Part model, mm, in its own coordinate system. A direction names the side the tool comes from. Give positions to 0.01 mm unless a question says otherwise; leave off trailing zeros. Order: outer loops, then holes, each group sorted by start corner. A loop starts at its lowest first (then second) coordinate and runs counter-clockwise, first axis right, second up. Notation, with made-up numbers: (9.25, -29) - (27.25, -29) arc R23 ccw to (27.25, -3) - close; hole circle Ø4 at (86, 65.25). An arc over 180 degrees is marked (long way). One line per item, written item: value.
```python
from build123d import *

# Parameters (mm, degrees)
SKETCH1_W           = 914.4
SKETCH1_H           = 203.2
BOSS_EXTRUDE1_DEPTH = 12.7
SKETCH2_W           = 914.4
SKETCH2_H           = 152.4
BOSS_EXTRUDE2_DEPTH = 12.7
SKETCH3_W           = 31.75
SKETCH3_H           = 419.1
BOSS_EXTRUDE3_DEPTH = 31.75
BOSS_EXTRUDE4_START = -914.4
SKETCH3_2_W         = 31.75
SKETCH3_2_H         = 419.1
BOSS_EXTRUDE4_DEPTH = 31.75


with BuildPart() as part:
    # Sketch1 → Boss-Extrude1 (new body)
    with BuildSketch(Plane(origin=(0, 0, 0), x_dir=(1, 0, 0), z_dir=(0, 1, 0))):
        with Locations((457.2, 101.6)):
            Rectangle(SKETCH1_W, SKETCH1_H)
    extrude(amount=BOSS_EXTRUDE1_DEPTH)



with BuildPart() as body_2:
    # Sketch2 → Boss-Extrude2 (new body)
    with BuildSketch(Plane(origin=(0, 215.9, 0), x_dir=(1, 0, 0), z_dir=(0, 1, 0))):
        with Locations((457.2, 127)):
            Rectangle(SKETCH2_W, SKETCH2_H)
    extrude(amount=BOSS_EXTRUDE2_DEPTH)


with BuildPart() as part_1:
    add(part.part)

    add(body_2.part)  # Boss-Extrude3 merges body 2
    # Sketch3 → Boss-Extrude3 (add)
    with BuildSketch(Plane(origin=(914.4, 0, 0), x_dir=(0, 0, -1), z_dir=(1, 0, 0))):
        with Locations((187.325, 19.05)):
            Rectangle(SKETCH3_W, SKETCH3_H)
        Polygon((0, 12.7), (0, -190.5), (31.75, -190.5), (31.75, 12.7), (82.55, 228.6), (50.8, 228.6), align=None)
    extrude(amount=-BOSS_EXTRUDE3_DEPTH)

    # Sketch3<2> → Boss-Extrude4 (add)
    with BuildSketch(Plane(origin=(914.4, 0, 0), x_dir=(0, 0, -1), z_dir=(1, 0, 0)).offset(BOSS_EXTRUDE4_START)):
        with Locations((187.325, 19.05)):
            Rectangle(SKETCH3_2_W, SKETCH3_2_H)
        Polygon((0, 12.7), (0, -190.5), (31.75, -190.5), (31.75, 12.7), (82.55, 228.6), (50.8, 228.6), align=None)
    extrude(amount=BOSS_EXTRUDE4_DEPTH)


solid = part_1.part
```
1) Cut at C-C, the plane z = -16. Give the cut face in (x, y), then the cut area to 3 significant figures.
Outcome:
outline: (0, -190.5) - (31.75, -190.5) - (31.75, 0) - (882.65, 0) - (882.65, -190.5) - (914.4, -190.5) - (914.4, 80.7) - (882.65, 80.7) - (882.65, 12.7) - (31.75, 12.7) - (31.75, 80.7) - (0, 80.7) - close
area: 28,000 mm^2
2) Cut at B-B, the plane z = -105.5. Give the cut face in (x, y).
Outcome:
outline: (0, 0) - (914.4, 0) - (914.4, 12.7) - (0, 12.7) - close; (0, 215.9) - (914.4, 215.9) - (914.4, 228.6) - (0, 228.6) - close
3) Cut at A-A, the plane x = 205. Give the cut face in (y, z).
Outcome:
outline: (0, -203.2) - (12.7, -203.2) - (12.7, 0) - (0, 0) - close; (215.9, -203.2) - (228.6, -203.2) - (228.6, -50.8) - (215.9, -50.8) - close
4) Pin check, flat tips, straight feed: pin 1 (12 mm diameter, centred on x = 379, z = -34, fed in from +Y); pin 2 (4 mm diameter, centred on x = 225, z = -164.5, fed in from -Y); pin 3 (6 mm diameter, centred on y = -43, z = -165.5, fed in from -X). Stop position of each tip, or through.
Outcome:
pin 1: stops at y = 12.7
pin 2: stops at y = 0
pin 3: passes through
5) Drill centre lines: line 1 along X through (y, z) = (-52.5, -189.5); line 2 along Y through (x, z) = (567.5, -152.5); line 3 along Y through (x, z) = (779, -21). Where is each one in solid material? Low to high. Write a range as from..to.
Outcome:
line 1: x = 0..31.75, 882.65..914.4
line 2: y = 0..12.7, 215.9..228.6
line 3: y = 0..12.7
6) Cut at D-D, the plane y = 154. Give the cut face in (x, z), then the cut area to 3 significant figures.
Outcome:
outline: (0, -203.2) - (31.75, -203.2) - (31.75, -171.45) - (0, -171.45) - close; (0, -65) - (31.75, -65) - (31.75, -33.25) - (0, -33.25) - close; (882.65, -203.2) - (914.4, -203.2) - (914.4, -171.45) - (882.65, -171.45) - close; (882.65, -65) - (914.4, -65) - (914.4, -33.25) - (882.65, -33.25) - close
area: 4,030 mm^2
7) Mould opens along Y. For faces 1 (the flat face through (16, -190.5, -187)), 2 (the flat face through (455, 1, 0)), 3 (the flat face through (899, 113, -171.45)) say: released by +Y, released by -Y, zero draft, split by the parting line, or undercut.
Outcome:
face 1: released by -Y
face 2: zero draft
face 3: undercut
8) Which spindle directions (+Z, -Z, +X, -X, +Y, -Y) get a long thin tool onto all of the face, cutting with end or side? Do faces 4 (the flat face through (16, -97, -171.45)), 5 (the flat face through (16, -190.5, -16)), 6 (the flat face through (15.65, 112.88, -55.32)), 7 (the flat face through (882.65, -94, -187)). Say none if no direction does.
Outcome:
face 4: +X, -X, -Y
face 5: +Z, -Z, +X, -X, -Y
face 6: +X, -X
face 7: +Z, -Z, -Y
